```python
from build123d import *

# Parameters (mm, degrees)
SKETCH1_W           = 30
SKETCH1_H           = 20
SKETCH1_R           = 2.5
BOSS_EXTRUDE1_DEPTH = 5
CUT_EXTRUDE1_DEPTH  = 5
SKETCH3_W           = 40
SKETCH3_H           = 50
BOSS_EXTRUDE2_DEPTH = 5
SKETCH4_W           = 5
SKETCH4_H           = 50
BOSS_EXTRUDE3_DEPTH = 30
SKETCH5_R           = 2.5
CUT_EXTRUDE2_DEPTH  = 20
FILLET1_R           = 10
FILLET2_R           = 10


with BuildPart() as part:
    # Sketch1 → Boss-Extrude1 (new body)
    with BuildSketch(Plane.XY):
        with Locations((-20.063803349, 8.047545841)):
            Rectangle(SKETCH1_W, SKETCH1_H)
        with Locations((-15.063803349, 8.047545841)):
            Circle(SKETCH1_R, mode=Mode.SUBTRACT)
    extrude(amount=BOSS_EXTRUDE1_DEPTH)

    # Sketch2 → Cut-Extrude1 (cut)
    with BuildSketch(Plane.XY.offset(5)):
        with BuildLine():
            ThreePointArc((-15.063803349, 18.047545841), (-7.992735537, 15.118613653), (-5.063803349, 8.047545841))
            Line((-5.063803349, 8.047545841), (-5.063803349, 18.047545841))
            Line((-5.063803349, 18.047545841), (-15.063803349, 18.047545841))
        make_face()
        with BuildLine():
            Line((-5.063803349, -1.952454159), (-5.063803349, 8.047545841))
            ThreePointArc((-5.063803349, 8.047545841), (-7.992735537, 0.976478029), (-15.063803349, -1.952454159))
            Line((-15.063803349, -1.952454159), (-5.063803349, -1.952454159))
        make_face()
    extrude(amount=-CUT_EXTRUDE1_DEPTH, mode=Mode.SUBTRACT)

    # Sketch3 → Boss-Extrude2 (add)
    with BuildSketch(Plane.ZY.offset(35.063803349)):
        with Locations((5, 8.047545841)):
            Rectangle(SKETCH3_W, SKETCH3_H)
    extrude(amount=BOSS_EXTRUDE2_DEPTH)

    # Sketch4 → Boss-Extrude3 (add)
    with BuildSketch(Plane(origin=(-35.063803349, 0, 0), x_dir=(0, 0, -1), z_dir=(1, 0, 0))):
        with Locations((12.5, 8.047545841)):
            Rectangle(SKETCH4_W, SKETCH4_H)
    extrude(amount=BOSS_EXTRUDE3_DEPTH)

    # Sketch5 → Cut-Extrude2 (cut)
    with BuildSketch(Plane.XY.offset(-10)):
        with Locations((-15.063803349, 28.047545841)):
            Circle(SKETCH5_R)
        with Locations((-15.063803349, -11.952454159)):
            Circle(SKETCH5_R)
    extrude(amount=-CUT_EXTRUDE2_DEPTH, mode=Mode.SUBTRACT)

    # Fillet1
    fillet1_edges = [part.edges().sort_by_distance(p)[0] for p in [
        (-5.063803349, 33.047545841, -12.5),
    ]]
    fillet(fillet1_edges, radius=FILLET1_R)

    # Fillet2
    fillet2_edges = [part.edges().sort_by_distance(p)[0] for p in [
        (-5.063803349, -16.952454159, -12.5),
    ]]
    fillet(fillet2_edges, radius=FILLET2_R)


solid = part.part
```
The listing builds one solid part. Answer for the finished solid, in the listing's coordinates (mm). A direction names the side the tool comes from. Coordinates: 2 decimals unless noted, no trailing zeros. Write each loop counter-clockwise with the first axis right and the second up, starting at its lowest first coordinate (ties: lowest second). Pieces come first, ordered by that corner, then holes. Notation, with made-up numbers: M -9,25.25 L 3,25.25 A13 cw 3,37.25 Z; hole C 19.25,43 d11. An arc over 180 degrees is marked long. Use a Markdown table: item, result. Add a question column.
1. Section B-B (y = 26.5) is taken. Give the vertices of the cut face in (x, z), plus the area to 3 significant figures.
2. For a pull along Y with two mould halves and no side action, classify faces 6 (the flat face through (-35.064, 8, 7)), 7 (the cylindrical face through (-15.606, 5.607, 2.465)), 8 (the cylindrical face through (-7.92, -13.95, -12.54)) as +Y half, -Y half, draft (parallel to the pull), parting line (faces both ways), or undercut.
3. Which of the six approach directions +Z, -Z, +X, -X, +Y, -Y give full straight-line access (tool end or side, diameter ignored) to faces 1 (the flat face through (-25, 18.048, 2)), 2 (the flat face through (-20, 8, 5)), 3 (the flat face through (-20, 8, 0)), 4 (the flat face through (-25, -1.952, 2)), 5 (the cylindrical face through (-15.389, 30.526, -12.465))?
4. Section A-A (x = -27) is taken. Give the vertices of the cut face in (y, z), plus the area to 3 significant figures.
5. Straight lines are drawn through the part: line 1 along Z through (x, y) = (-26.5, 10.5); line 2 along Y through (x, z) = (-16, -12); line 3 along Z through (x, y) = (-26.5, -12). For each, find the intervals that lie inside material, in ascending order. Write a range as [from, to].
6. Section C-C (x = -13.5) is taken. Give the vertices of the cut face in (y, z), plus the area to 3 significant figures.
7. Section D-D (y = 19) is taken. Give the vertices of the cut face in (x, z), plus the area to 3 significant figures.
8. Given P1, Ø15, axis at x = -19.5, y = -4, coming from the +Z side; P2, Ø4, axis at x = -19.5, z = 3.5, coming from the +Y side; P3, Ø1.5, axis at y = 5, z = -7, coming from the +X side; P4, Ø4, axis at x = -15.06, y = 28.05, coming from the +Z side, each flat-ended and moving along its own axis, determine where each tip first touches the part or whether it passes through.
Data:
| question | item | result |
|---|---|---|
| 1 | outline | M -40.06,-15 L -17.03,-15 L -17.03,-10 L -35.06,-10 L -35.06,25 L -40.06,25 Z; M -13.1,-15 L -5.68,-15 L -5.68,-10 L -13.1,-10 Z |
| 1 | area | 327 mm2 |
| 2 | face 6 | draft |
| 2 | face 7 | undercut |
| 2 | face 8 | -Y half |
| 3 | face 1 | +Z, +X, +Y |
| 3 | face 2 | +Z, +X, +Y, -Y |
| 3 | face 3 | +X, +Y, -Y |
| 3 | face 4 | +Z, +X, -Y |
| 3 | face 5 | +Z, -Z |
| 4 | outline | M -16.95,-15 L 33.05,-15 L 33.05,-10 L -16.95,-10 Z; M -1.95,0 L 18.05,0 L 18.05,5 L -1.95,5 Z |
| 4 | area | 350 mm2 |
| 5 | line 1 | z = [-15, -10], [0, 5] |
| 5 | line 2 | y = [-16.95, -14.27], [-9.63, 25.73], [30.37, 33.05] |
| 5 | line 3 | z = [-15, -10] |
| 6 | outline | M -16.83,-15 L -13.9,-15 L -13.9,-10 L -16.83,-10 Z; M -10,-15 L 26.1,-15 L 26.1,-10 L -10,-10 Z; M -1.83,0 L 6.1,0 L 6.1,5 L -1.83,5 Z; M 10,0 L 17.92,0 L 17.92,5 L 10,5 Z; M 30,-15 L 32.92,-15 L 32.92,-10 L 30,-10 Z |
| 6 | area | 289 mm2 |
| 7 | outline | M -40.06,-15 L -5.06,-15 L -5.06,-10 L -35.06,-10 L -35.06,25 L -40.06,25 Z |
| 7 | area | 350 mm2 |
| 8 | P1 | stops at z = 5 |
| 8 | P2 | stops at y = 18.05 |
| 8 | P3 | stops at x = -35.06 |
| 8 | P4 | passes through |
